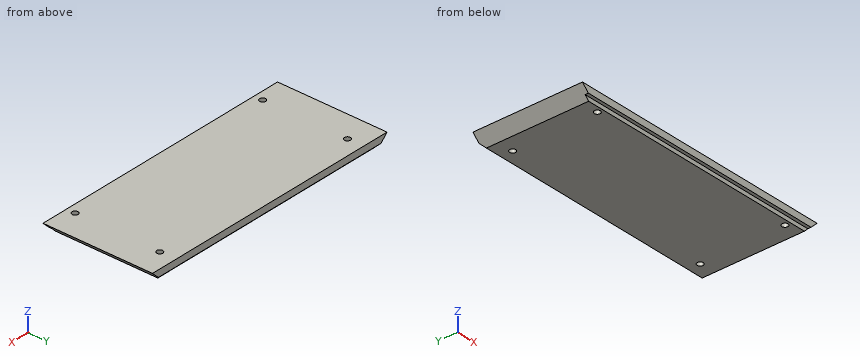
from build123d import *

# Parameters (mm, degrees)
SKETCH1_W           = 200
SKETCH1_H           = 84
SKETCH1_R           = 2.25
BOSS_EXTRUDE1_DEPTH = 5
SKETCH2_W           = 200
SKETCH2_H           = 79
SKETCH2_R           = 2.25
BOSS_EXTRUDE2_DEPTH = 3
CHAMFER1_SIZE       = 8
CHAMFER3_SIZE       = 3
SKETCH3_W           = 7.071067812
SKETCH3_H           = 2.6
CUT_EXTRUDE1_DEPTH  = 234.034075139


with BuildPart() as part:
    # Sketch1 → Boss-Extrude1 (new body)
    with BuildSketch(Plane.XY):
        with Locations((100, 42)):
            Rectangle(SKETCH1_W, SKETCH1_H)
        with Locations((20, 9)):
            Circle(SKETCH1_R, mode=Mode.SUBTRACT)
        with Locations(Location((180, 9, 0), (0, 0, 180))):
            Circle(SKETCH1_R, mode=Mode.SUBTRACT)
        with Locations((20, 72)):
            Circle(SKETCH1_R, mode=Mode.SUBTRACT)
        with Locations(Location((180, 72, 0), (0, 0, 180))):
            Circle(SKETCH1_R, mode=Mode.SUBTRACT)
    extrude(amount=-BOSS_EXTRUDE1_DEPTH)

    # Sketch2 → Boss-Extrude2 (add)
    with BuildSketch(Plane(origin=(0, 0, -5), x_dir=(-1, 0, 0), z_dir=(0, 0, -1))):
        with Locations((-100, 44.5)):
            Rectangle(SKETCH2_W, SKETCH2_H)
        with Locations(Location((-20, 9, 0), (0, 0, 180))):
            Circle(SKETCH2_R, mode=Mode.SUBTRACT)
        with Locations((-180, 9)):
            Circle(SKETCH2_R, mode=Mode.SUBTRACT)
        with Locations(Location((-20, 72, 0), (0, 0, 180))):
            Circle(SKETCH2_R, mode=Mode.SUBTRACT)
        with Locations((-180, 72)):
            Circle(SKETCH2_R, mode=Mode.SUBTRACT)
    extrude(amount=BOSS_EXTRUDE2_DEPTH)

    # Chamfer1
    # the kernel refuses this chamfer: 8 mm, written as the material it takes off along each edge
    with BuildSketch(Plane(origin=(200, -15.573463904, -8), x_dir=(-0.9996219169112968, 0, -0.027495876610586296), z_dir=(0, 1, 0)), Plane(origin=(0, 104.573463904, -8), x_dir=(0.9996219169112968, 0, -0.027495876610586275), z_dir=(0, -1, 0))) as chamfer1_piece_1:
        Polygon((CHAMFER1_SIZE * 0.999621916911, CHAMFER1_SIZE * 0.0274958766106), (-CHAMFER1_SIZE * 0.0274958766106, CHAMFER1_SIZE * 0.999621916911), (0, 0), align=None)
    extrude(amount=120.146927807, mode=Mode.SUBTRACT)

    # Chamfer3
    chamfer3_edges = [part.edges().sort_by_distance(p)[0] for p in [
        (100, 84, -8),
    ]]
    chamfer(chamfer3_edges, length=CHAMFER3_SIZE)

    # Sketch3 → Cut-Extrude1 (cut, through all, along a direction that is not the sketch's normal)
    with BuildSketch(Plane(origin=(100, 0, -100), x_dir=(-0.7071067811865452, 0, -0.7071067811865498), z_dir=(0.7071067811865498, 0, -0.7071067811865452))):
        with Locations((-137.885822331, 1.3)):
            Rectangle(SKETCH3_W, SKETCH3_H)
    extrude(amount=-CUT_EXTRUDE1_DEPTH, dir=(1, 0, 0), mode=Mode.SUBTRACT)


solid = part.part
The model under review builds one solid part; all positions refer to its coordinate system, in mm. Give positions to 0.01 mm unless a question says otherwise; leave off trailing zeros. Write each loop counter-clockwise with the first axis right and the second up, starting at its lowest first coordinate (ties: lowest second). Pieces come first, ordered by that corner, then holes.
1. Add section D-D, the plane x = 58. Write out the cut boundary in (y, z), plus the area to 4 significant figures.
2. Add section B-B, the plane z = -2.25. Write out the cut boundary in (x, y), plus the area to 3 significant figures.
3. For P1, Ø4, axis at x = 20, y = 9, coming from the +Z side; P2, Ø1.5, axis at y = 72, z = -2, coming from the -X side; P3, Ø1.2, axis at x = 123, y = 3.5, coming from the -Z side; P4, Ø1.5, axis at x = 102.5, z = -6, coming from the -Y side, all flat-tipped, find the tip position at first contact; note any pin that passes through.
4. Wall thickness on L1, parallel to Y at x = 180, z = -2.35; L2, parallel to X at y = 72, z = -5.9; L3, parallel to Y at x = 20, z = -6.15: over which ranges is each line inside the solid? List them lowest first.
5. Add section C-C, the plane x = 20. Write out the cut boundary in (y, z), plus the area to 4 significant figures.
6. Add section A-A, the plane y = 72. Write out the cut boundary in (x, z).
Worked answers:
1. outline: (2.6, -5) - (5, -5) - (5, -8) - (81, -8) - (84, -5) - (84, 0) - (2.6, 0) - close
1. area: 639.5 mm2
2. outline: (2.25, 2.6) - (197.75, 2.6) - (197.75, 84) - (2.25, 84) - close; hole circle Ø4.5 at (20, 9); hole circle Ø4.5 at (20, 72); hole circle Ø4.5 at (180, 9); hole circle Ø4.5 at (180, 72)
2. area: 15,900 mm2
3. P1: passes through
3. P2: stops at x = 1.25
3. P3: stops at z = -5
3. P4: stops at y = 5
4. L1: y = 2.6 to 6.75, 11.25 to 69.75, 74.25 to 84
4. L2: x = 5.9 to 17.75, 22.25 to 177.75, 182.25 to 194.1
4. L3: y = 5 to 6.75, 11.25 to 69.75, 74.25 to 82.85
5. outline: (2.6, -5) - (5, -5) - (5, -8) - (6.75, -8) - (6.75, 0) - (2.6, 0) - close; (11.25, -8) - (69.75, -8) - (69.75, 0) - (11.25, 0) - close; (74.25, -8) - (81, -8) - (84, -5) - (84, 0) - (74.25, 0) - close
5. area: 567.5 mm2
6. outline: (0, 0) - (8, -8) - (17.75, -8) - (17.75, 0) - close; (22.25, -8) - (177.75, -8) - (177.75, 0) - (22.25, 0) - close; (182.25, -8) - (192, -8) - (200, 0) - (182.25, 0) - close
